from build123d import *

# Parameters (mm, degrees)
F1_DEPTH      = 25
F1_TAPER      = 3
F1_DEPTH_BACK = 58.2
F1_TAPER_BACK = -3
F2_R          = 10.5652829809
F3_T          = -2.5


with BuildPart() as f1:
    # F0 (on Top) → F1 (new body, two sides)
    with BuildSketch(Plane.XY) as f1_sk:
        Polygon((-20.5419126951, -42.6557212379), (20.5419126951, -42.6557212379), (46.1572588473, -10.5350931276), (37.0152476509, 29.5186749845), (0, 47.3442787621), (-37.0152476509, 29.5186749845), (-46.1572588473, -10.5350931276), align=None)
    extrude(amount=F1_DEPTH, taper=F1_TAPER)
    extrude(f1_sk.sketch, amount=-F1_DEPTH_BACK, taper=F1_TAPER_BACK)

    # F2
    f2_edges = [f1.edges().sort_by_distance(p)[0] for p in [
        (-32.325234, -25.778514, 25),
        (0, -41.345527, 25),
        (32.325234, -25.778514, 25),
        (40.308908, 9.200245, 25),
        (17.939152, 37.251032, 25),
        (-17.939152, 37.251032, 25),
        (-40.308908, 9.200245, 25),
    ]]
    fillet(f2_edges, radius=F2_R)

    # F3
    f3_openings = [f1.faces().sort_by_distance(p)[0] for p in [
        (0, 0, -58.2),
    ]]
    offset(amount=F3_T, openings=f3_openings)


solid = f1.part
Geometry: final body of the model. Coordinates: model frame, mm. A direction names the side the tool comes from. Round coordinates to 2 decimals unless told otherwise and drop trailing zeros. Loops run counter-clockwise (first coordinate to the right, second up) from the corner with the lowest first, then second, coordinate; pieces in that order, holes last. Notation, with made-up numbers: M 34,72.5 L 40,72.5 A28 cw 40,91.5 Z; hole C -4.5,75 d7. An arc over 180 degrees is marked long. Put each result on its own line as item: value. Start each with the question number.
(1) Section query A-A (z = 11). Return loops of the section in (x, y) (3 decimals).
(2) Set-up query: faces 4 (the face through (-0.291, -41.315, -22.183)), 5 (the face through (-29.93, -24.23, 22.18)). Return all of +Z, -Z, +X, -X, +Y, -Y with unobstructed straight access to the full face (end or side cutting, diameter ignored); none if empty.
(3) Contact query for flat-ended pins moving along their axis: pin 1 Ø12 at (y, z) = (-14, -13) entering from -X; pin 2 Ø3 at (x, y) = (-6, -7) entering from -Z; pin 3 Ø8 at (y, z) = (0, -7) entering from -X. Output: stop coordinate, or through.
(4) Draft query along X for faces 1 (the face through (-40.214, 9.477, -22.183)), 2 (the face through (-42.648, 10.05, -22.118)), 3 (the face through (0, 2, 25)). Return one class per face: +X half, -X half, draft (parallel to the pull), parting line (faces both ways), or undercut.
(5) Material intervals for line 1 along Z through (x, y) = (-15.5, 13.5); line 2 along X through (y, z) = (18.5, 5.5); line 3 along X through (y, z) = (-40, -18), sorted ascending. Write a range as [from, to].
Findings below:
1. outline: M -45.533,-10.393 L -20.264,-42.079 L 20.264,-42.079 L 45.533,-10.393 L 36.515,29.12 L 0,46.704 L -36.515,29.12 Z; hole M -42.825,-9.774 L -19.059,-39.576 L 19.059,-39.576 L 42.825,-9.774 L 34.343,27.387 L 0,43.926 L -34.343,27.387 Z
2. face 4: -Z
2. face 5: +Z, -X, -Y
3. pin 1: stops at x = -47.18
3. pin 2: stops at z = 22.5
3. pin 3: stops at x = -45.07
4. face 1: undercut
4. face 2: -X half
4. face 3: draft
5. line 1: z = [22.5, 25]
5. line 2: x = [-39.23, -36.67], [36.67, 39.23]
5. line 3: x = [-23.87, -20.66], [20.66, 23.87]
